```python
from build123d import *

# Parameters (mm, degrees)
F0_R     = 14.2875
F1_DEPTH = 25.4
F2_DEPTH = 105.156
F3_DEPTH = 87.884


with BuildPart() as f1:
    # F0 (on Front) → F1 (new body)
    with BuildSketch(Plane.XZ):
        with BuildLine():
            ThreePointArc((5.4312411777, -28.0540949644), (22.0423268015, -18.1842364199), (28.575, 0))
            ThreePointArc((28.575, 0), (22.0423268015, 18.1842364199), (5.4312411777, 28.0540949644))
            ThreePointArc((5.4312411777, 28.0540949644), (-28.575, 0), (5.4312411777, -28.0540949644))
        make_face()
        with BuildLine():
            ThreePointArc((-13.4703841816, 4.7625), (0, 14.2875), (13.4703841816, 4.7625))
            Line((13.4703841816, 4.7625), (19.05, 4.7625))
            Line((19.05, 4.7625), (19.05, -4.7625))
            Line((19.05, -4.7625), (13.4703841816, -4.7625))
            ThreePointArc((13.4703841816, -4.7625), (0, -14.2875), (-13.4703841816, -4.7625))
            Line((-13.4703841816, -4.7625), (-19.05, -4.7625))
            Line((-19.05, -4.7625), (-19.05, 4.7625))
            Line((-19.05, 4.7625), (-13.4703841816, 4.7625))
        make_face(mode=Mode.SUBTRACT)
        with BuildLine():
            ThreePointArc((69.1631999291, 0), (64.8080844634, 12.1228242799), (53.7340273808, 18.7027299762))
            ThreePointArc((53.7340273808, 18.7027299762), (31.0631999291, 0), (53.7340273808, -18.7027299762))
            ThreePointArc((53.7340273808, -18.7027299762), (64.8080844634, -12.1228242799), (69.1631999291, 0))
        make_face()
        with Locations((50.1131999291, 0)):
            Circle(F0_R, mode=Mode.SUBTRACT)
        with BuildLine():
            ThreePointArc((5.4312411777, 28.0540949644), (22.0423268015, 18.1842364199), (28.575, 0))
            ThreePointArc((28.575, 0), (22.0423268015, -18.1842364199), (5.4312411777, -28.0540949644))
            Line((5.4312411777, -28.0540949644), (53.7340273808, -18.7027299762))
            ThreePointArc((53.7340273808, -18.7027299762), (31.0631999291, 0), (53.7340273808, 18.7027299762))
            Line((53.7340273808, 18.7027299762), (5.4312411777, 28.0540949644))
        make_face()
        with BuildLine():
            ThreePointArc((-13.4703841816, -4.7625), (-14.2875, 0), (-13.4703841816, 4.7625))
            Line((-13.4703841816, 4.7625), (-19.05, 4.7625))
            Line((-19.05, 4.7625), (-19.05, -4.7625))
            Line((-19.05, -4.7625), (-13.4703841816, -4.7625))
        make_face()
    extrude(amount=F1_DEPTH)

    # F0 (on Front) → F2 (join)
    with BuildSketch(Plane.XZ):
        with BuildLine():
            ThreePointArc((5.4312411777, -28.0540949644), (22.0423268015, -18.1842364199), (28.575, 0))
            ThreePointArc((28.575, 0), (22.0423268015, 18.1842364199), (5.4312411777, 28.0540949644))
            ThreePointArc((5.4312411777, 28.0540949644), (-28.575, 0), (5.4312411777, -28.0540949644))
        make_face()
        with BuildLine():
            ThreePointArc((-13.4703841816, 4.7625), (0, 14.2875), (13.4703841816, 4.7625))
            Line((13.4703841816, 4.7625), (19.05, 4.7625))
            Line((19.05, 4.7625), (19.05, -4.7625))
            Line((19.05, -4.7625), (13.4703841816, -4.7625))
            ThreePointArc((13.4703841816, -4.7625), (0, -14.2875), (-13.4703841816, -4.7625))
            Line((-13.4703841816, -4.7625), (-19.05, -4.7625))
            Line((-19.05, -4.7625), (-19.05, 4.7625))
            Line((-19.05, 4.7625), (-13.4703841816, 4.7625))
        make_face(mode=Mode.SUBTRACT)
    extrude(amount=F2_DEPTH)

    # F0 (on Front) → F3 (join)
    with BuildSketch(Plane.XZ):
        with BuildLine():
            ThreePointArc((69.1631999291, 0), (64.8080844634, 12.1228242799), (53.7340273808, 18.7027299762))
            ThreePointArc((53.7340273808, 18.7027299762), (31.0631999291, 0), (53.7340273808, -18.7027299762))
            ThreePointArc((53.7340273808, -18.7027299762), (64.8080844634, -12.1228242799), (69.1631999291, 0))
        make_face()
        with Locations((50.1131999291, 0)):
            Circle(F0_R, mode=Mode.SUBTRACT)
    extrude(amount=F3_DEPTH)


solid = f1.part
```
Design review of the part built by this model. Coordinates are the model's own, in mm. A direction names the side the tool comes from. Coordinates: 2 decimals unless noted, no trailing zeros. Loops run counter-clockwise (first coordinate to the right, second up) from the corner with the lowest first, then second, coordinate; pieces in that order, holes last. Notation, with made-up numbers: (21.25, -35) -> (59.25, -35) arc R29 cw to (59.25, -11) -> close; hole circle Ø1 at (30.25, -25.5). An arc over 180 degrees is marked (long way). Answer as a JSON object with one key per item and string values.
Q1. Take a section at A-A on y = -52. Give the number of separate pieces and of enclosed holes in the cut face, plus the area to 3 significant figures.
Answer block:
{"separate pieces": "2", "enclosed holes": "2", "area": "2,330 mm^2"}
Q2. To check wall thickness, follow L1, parallel to Z at x = 51, y = -30.5; L2, parallel to X at y = -42, z = 12.5; L3, parallel to X at y = -36.5, z = 3.5. State the ranges of each line that lie inside material, in increasing order.
Answer block:
{"L1": "z = -19.03 to -14.26, 14.26 to 19.03", "L2": "x = -25.7 to -6.92, 6.92 to 25.7, 35.74 to 43.19, 57.03 to 64.49", "L3": "x = -28.36 to -19.05, 19.05 to 28.36, 31.39 to 36.26, 63.97 to 68.84"}
Q3. The part is to be moulded in two halves that separate along Z. For faces 1 (the cylindrical face through (-28.564, -51.842, 0.779)), 2 (the flat face through (16, -52, -4.762)), 3 (the flat face through (-16, -65, 4.762)), 4 (the flat face through (-13, -105.156, 7)), say which applies: +Z half, -Z half, draft (parallel to the pull), parting line (faces both ways), or undercut.
Answer block:
{"face 1": "parting line", "face 2": "undercut", "face 3": "undercut", "face 4": "draft"}
Q4. Take a section at C-C on x = 0. Give the boundary of the cut face in (y, z) (1 decimal).
Answer block:
{"outline": "(-105.2, -28.6) -> (0, -28.6) -> (0, -14.3) -> (-105.2, -14.3) -> close; (-105.2, 14.3) -> (0, 14.3) -> (0, 28.6) -> (-105.2, 28.6) -> close"}
Q5. Clearance check with flat-ended pins moving along their axes: pin 1 Ø3 at (x, y) = (-15, -66.5) entering from +Z; pin 2 Ø5 at (y, z) = (-38.5, -22.5) entering from +X; pin 3 Ø8 at (x, z) = (-15, -11.5) entering from +Y; pin 4 Ø4 at (y, z) = (-29, -21) entering from -X. State where each tip first meets the part, or that it passes through.
Answer block:
{"pin 1": "stops at z = 25.18", "pin 2": "stops at x = 20.41", "pin 3": "stops at y = 0", "pin 4": "stops at x = -21.34"}
Q6. Tool access review of faces 5 (the flat face through (20, 0, 0)), 6 (the flat face through (19.05, -52, 0)), 7 (the flat face through (52.8, -87.884, 14.2)), 8 (the flat face through (29.921, -12.522, 23.313)), 9 (the flat face through (29, -25.4, 0)): name each direction out of +Z, -Z, +X, -X, +Y, -Y from which nothing blocks a thin tool from reaching the whole face with its end or side.
Answer block:
{"face 5": "+Z, -Z, +X, -X, +Y", "face 6": "+Y, -Y", "face 7": "+Z, -Z, +X, -Y", "face 8": "+Z, +X, +Y, -Y", "face 9": "-Y"}
